```python
from build123d import *

# Parameters (mm, degrees)
F1_DEPTH = 12.7
F2_R     = 3.175
F3_DEPTH = 25.4
F4_R     = 3.175
F5_DEPTH = 25.4


with BuildPart() as f1:
    # F0 (on Right) → F1 (new body)
    with BuildSketch(Plane.YZ):
        with BuildLine():
            Line((0, 25.4), (0, 3.048))
            ThreePointArc((0, 3.048), (0.892739, 0.892739), (3.048, 0))
            Line((3.048, 0), (25.4, 0))
            Line((25.4, 0), (25.4, 1.524))
            Line((25.4, 1.524), (4.572, 1.524))
            ThreePointArc((4.572, 1.524), (2.416739, 2.416739), (1.524, 4.572))
            Line((1.524, 4.572), (1.524, 25.4))
            Line((1.524, 25.4), (0, 25.4))
        make_face()
    extrude(amount=F1_DEPTH)

    # F2 (on face) → F3 (cut)
    with BuildSketch(Plane(origin=(0, 1.524, 0), x_dir=(-1, 0, 0), z_dir=(0, 1, 0))):
        with Locations((-6.35, 19.05)):
            Circle(F2_R)
    extrude(amount=-F3_DEPTH, mode=Mode.SUBTRACT)

    # F4 (on face) → F5 (cut)
    with BuildSketch(Plane(origin=(0, 0, 0), x_dir=(1, 0, 0), z_dir=(0, 0, -1))):
        with Locations((6.35, -19.05)):
            Circle(F4_R)
    extrude(amount=-F5_DEPTH, mode=Mode.SUBTRACT)


solid = f1.part
```
Could you check a few things on this model? Use its own coordinates, in mm. A direction names the side the tool comes from. Coordinates: 2 decimals unless noted, no trailing zeros. Write each loop counter-clockwise with the first axis right and the second up, starting at its lowest first coordinate (ties: lowest second). Pieces come first, ordered by that corner, then holes. Notation, with made-up numbers: (38.5, 59) -> (74.5, 59) arc R29 cw to (74.5, 92) -> close; hole circle Ø9 at (69.25, 8). An arc over 180 degrees is marked (long way). Return JSON: item names as keys, results as strings.
(1) Imagine slicing it at D-D, the plane x = 1.75. Please give me the cut outline in (y, z), then the cut area to 3 significant figures.
Numbers:
{"outline": "(0, 3.05) arc R3.05 ccw to (3.05, 0) -> (25.4, 0) -> (25.4, 1.52) -> (4.57, 1.52) arc R3.05 cw to (1.52, 4.57) -> (1.52, 25.4) -> (0, 25.4) -> close", "area": "75.1 mm2"}
(2) We'd pull the mould along Y, two halves only. Please class faces 1 (the flat face through (6, 14, 0)), 2 (the flat face through (6, 0, 14)), 3 (the cylindrical face through (3.18, 18.91, 0.75)), 4 (the cylindrical face through (6.261, 2.441, 2.393)): +Y half, -Y half, draft (parallel to the pull), parting line (faces both ways), or undercut.
Numbers:
{"face 1": "draft", "face 2": "-Y half", "face 3": "undercut", "face 4": "+Y half"}
(3) Imagine slicing it at B-B, the plane x = 6.35. Please give me the cut outline in (y, z) (3 decimals).
Numbers:
{"outline": "(0, 3.048) arc R3.048 ccw to (3.048, 0) -> (15.875, 0) -> (15.875, 1.524) -> (4.572, 1.524) arc R3.048 cw to (1.524, 4.572) -> (1.524, 15.875) -> (0, 15.875) -> close; (0, 22.225) -> (1.524, 22.225) -> (1.524, 25.4) -> (0, 25.4) -> close; (22.225, 0) -> (25.4, 0) -> (25.4, 1.524) -> (22.225, 1.524) -> close"}
(4) I'm going to push flat-ended pins straight in: pin 1 (5.5 mm diameter, centred on x = 6.35, y = 19.05, fed in from -Z); pin 2 (5 mm diameter, centred on x = 8, y = 9, fed in from +Z); pin 3 (4 mm diameter, centred on x = 5, z = 18.5, fed in from +Y); pin 4 (5 mm diameter, centred on x = 4, z = 21, fed in from -Y). Where does each tip first touch, or does it pass through?
Numbers:
{"pin 1": "passes through", "pin 2": "stops at z = 1.52", "pin 3": "stops at y = 1.52", "pin 4": "stops at y = 0"}
(5) Imagine slicing it at A-A, the plane z = 19.05. Please give me the cut outline in (x, y) (3 decimals).
Numbers:
{"outline": "(0, 0) -> (3.175, 0) -> (3.175, 1.524) -> (0, 1.524) -> close; (9.525, 0) -> (12.7, 0) -> (12.7, 1.524) -> (9.525, 1.524) -> close"}
(6) I need wall thicknesses on L1, parallel to X at y = 19.05, z = 1.2 (3 decimals); L2, parallel to Z at x = 10, y = 15.75. Which ranges of each line are inside material? Lowest first, please.
Numbers:
{"L1": "x = 0 to 3.175, 9.525 to 12.7", "L2": "z = 0 to 1.52"}
(7) Which directions (+Z, -Z, +X, -X, +Y, -Y) give clear straight access to the entire face, cutting with the end or side of a thin tool? Please do faces 5 (the flat face through (6, 15, 1.524)), 6 (the cylindrical face through (7.04, 0.77, 15.95)).
Numbers:
{"face 5": "+Z, +X, -X, +Y", "face 6": "+Y, -Y"}
